Job drawing, mm, ordinate dimensions from the low corner. One solid piece. Give positions to 0.01 mm unless a question says otherwise; leave off trailing zeros. Loops run counter-clockwise (first coordinate to the right, second up) from the corner with the lowest first, then second, coordinate; pieces in that order, holes last. Notation, with made-up numbers: M 81,-23.5 L 98,-23.5 A34 ccw 98,11.5 Z; hole C 59.25,10.5 d4. An arc over 180 degrees is marked long. Answer in a Markdown table with one row per item.
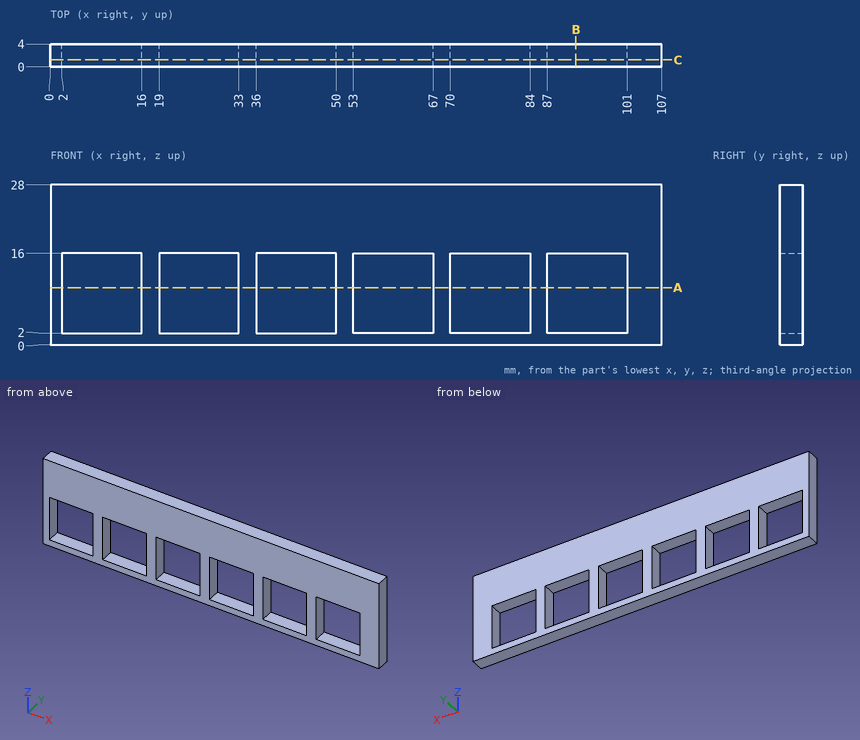
(1) Saw through at A-A (z = 10). Write the cut outline in (x, y), plus the area to 3 significant figures.
Recorded:
| item | result |
|---|---|
| outline | M 0,0 L 2,0 L 2,4 L 0,4 Z; M 16,0 L 19,0 L 19,4 L 16,4 Z; M 33,0 L 36,0 L 36,4 L 33,4 Z; M 50,0 L 53,0 L 53,4 L 50,4 Z; M 67,0 L 70,0 L 70,4 L 67,4 Z; M 84,0 L 87,0 L 87,4 L 84,4 Z; M 101,0 L 107,0 L 107,4 L 101,4 Z |
| area | 92.0 mm^2 |
(2) Drill centre line: line 1 along Z through (x, y) = (83, 1.5). Where is it in solid material? Low to high.
Recorded:
| item | result |
|---|---|
| line 1 | z = 0 to 2, 16 to 28 |
(3) Saw through at C-C (y = 1.2). Write the cut outline in (x, z), plus the area to 3 significant figures.
Recorded:
| item | result |
|---|---|
| outline | M 0,0 L 107,0 L 107,28 L 0,28 Z; hole M 2,2 L 16,2 L 16,16 L 2,16 Z; hole M 19,2 L 33,2 L 33,16 L 19,16 Z; hole M 36,2 L 50,2 L 50,16 L 36,16 Z; hole M 53,2 L 67,2 L 67,16 L 53,16 Z; hole M 70,2 L 84,2 L 84,16 L 70,16 Z; hole M 87,2 L 101,2 L 101,16 L 87,16 Z |
| area | 1,820 mm^2 |
(4) Saw through at B-B (x = 92). Write the cut outline in (y, z), plus the area to 3 significant figures.
Recorded:
| item | result |
|---|---|
| outline | M 0,0 L 4,0 L 4,2 L 0,2 Z; M 0,16 L 4,16 L 4,28 L 0,28 Z |
| area | 56.0 mm^2 |
